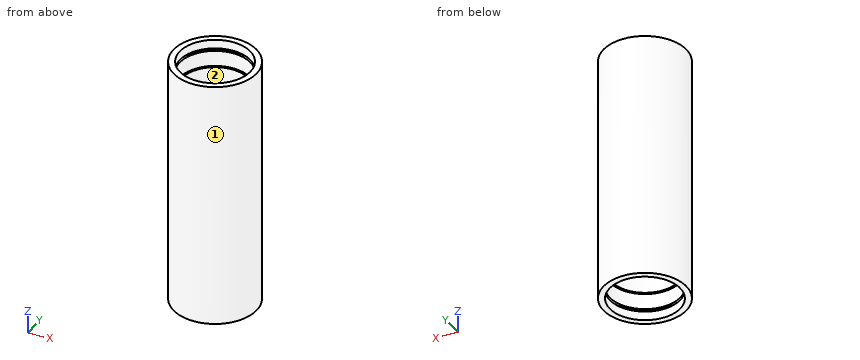
from build123d import *

# Parameters (mm, degrees)
SKETCH1_R           = 50
BOSS_EXTRUDE1_DEPTH = 150
SKETCH2_R           = 42.5
CUT_EXTRUDE1_DEPTH  = 33
SKETCH3_R           = 40
CUT_EXTRUDE2_DEPTH  = 277.204634284
SKETCH4_W           = 10
SKETCH4_H           = 3.2


with BuildPart() as part:
    # Sketch1 → Boss-Extrude1 (new, symmetric)
    with BuildSketch(Plane.XY):
        Circle(SKETCH1_R)
    extrude(amount=BOSS_EXTRUDE1_DEPTH, both=True)

    # Sketch2 → Cut-Extrude1 (cut)
    with BuildSketch(Plane.XY.offset(150)):
        Circle(SKETCH2_R)
    cut_extrude1 = extrude(amount=-CUT_EXTRUDE1_DEPTH, mode=Mode.SUBTRACT)

    # Sketch3 → Cut-Extrude2 (cut, through all)
    with BuildSketch(Plane.XY.offset(117)):
        Circle(SKETCH3_R)
    cut_extrude2 = extrude(amount=-CUT_EXTRUDE2_DEPTH, mode=Mode.SUBTRACT)

    # Sketch4 → Cut-Revolve1 (revolve, cut)
    with BuildSketch(Plane(origin=(0, 0, 0), x_dir=(1, 0, 0), z_dir=(0, 1, 0))):
        with Locations((40.5, -137.6)):
            Rectangle(SKETCH4_W, SKETCH4_H)
    cut_revolve1 = revolve(axis=Axis((0, 0, 150), (0, 0, 1)), mode=Mode.SUBTRACT)

    # Mirror1: Cut-Extrude1, Cut-Extrude2, Cut-Revolve1 across plane
    add(cut_extrude1.mirror(Plane.XY), mode=Mode.SUBTRACT)
    add(cut_extrude2.mirror(Plane.XY), mode=Mode.SUBTRACT)
    add(cut_revolve1.mirror(Plane.XY), mode=Mode.SUBTRACT)


solid = part.part
Geometry check sheet. Reference: the model listing, model coordinates, mm. Face numbers are marked on the shaded views. Round coordinates to 2 decimals unless told otherwise and drop trailing zeros. Write each loop counter-clockwise with the first axis right and the second up, starting at its lowest first coordinate (ties: lowest second). Pieces come first, ordered by that corner, then holes.
Item 1: Material ranges on line 1 along Z through (x, y) = (-42.5, 6); line 2 along Y through (x, z) = (0, -145); line 3 along Y through (x, z) = (0, 16.5), recorded low to high.
Determined:
line 1: z = -150 to -139.2, -136 to 136, 139.2 to 150
line 2: y = -50 to -42.5, 42.5 to 50
line 3: y = -50 to -40, 40 to 50
Item 2: Section check C-C (z = 30.5). Record the boundary of the cut face in (x, y), plus the area to 3 significant figures.
Determined:
outline: circle Ø100 at (0, 0); hole circle Ø80 at (0, 0)
area: 2,830 mm2
Item 3: Mould release check, pull along X, two halves, no side actions. Record for the marked faces 1 and 2: +X half, -X half, draft (parallel to the pull), parting line (faces both ways), or undercut.
Determined:
face 1: parting line
face 2: undercut
Item 4: Go/stop test with flat-tipped pins: pin 1 Ø12 at (y, z) = (-7, 59) entering from -X; pin 2 Ø8 at (x, z) = (-12, 14) entering from +Y; pin 3 Ø6 at (y, z) = (33, -77.5) entering from +X. Record where each tip stops, or that it passes through.
Determined:
pin 1: stops at x = -49.99
pin 2: stops at y = 49.36
pin 3: stops at x = 40
